For this review, take the finished solid that the model builds, in its own axes (mm). Face numbers are marked on the shaded views. A direction names the side the tool comes from. Round coordinates to 2 decimals unless told otherwise and drop trailing zeros. Write each loop counter-clockwise with the first axis right and the second up, starting at its lowest first coordinate (ties: lowest second). Pieces come first, ordered by that corner, then holes. Notation, with made-up numbers: M 33,-2.5 L 55,-2.5 A18 ccw 55,26.5 Z; hole C 64.25,-35.75 d5. An arc over 180 degrees is marked long. One line per question, with ' | ' between items.
```python
from build123d import *

# Parameters (mm, degrees)
EXTRUSION1_DEPTH = 28.5


with BuildPart() as part:
    # Esquisse1 → Révolution1 (revolve)
    with BuildSketch(Plane.XY):
        Polygon((-2.5, 19.6), (-2.5, 26), (-0.5, 26), (-0.5, 23.6), (2.5, 23.6), (2.5, 30), (20, 30), (20, 23.6), (23, 23.6), (23, 26), (25, 26), (25, 4), (10, 4), (10, 19.6), align=None)
    revolve(axis=Axis((10, 0, 0), (1, 0, 0)))

    # Esquisse2 → Extrusion1 (cut, through all)
    with BuildSketch(Plane(origin=(25, 0, 0), x_dir=(0, 0, -1), z_dir=(1, 0, 0))):
        with BuildLine():
            Line((17.944358445, 3), (-17.944358445, 3))
            ThreePointArc((-17.944358445, 3), (-19.127003214, 3.577312972), (-19.399306427, 4.864864865))
            ThreePointArc((-19.399306427, 4.864864865), (0, 20), (19.399306427, 4.864864865))
            ThreePointArc((19.399306427, 4.864864865), (19.127003214, 3.577312972), (17.944358445, 3))
        make_face()
    extrude(amount=-EXTRUSION1_DEPTH, mode=Mode.SUBTRACT)


solid = part.part
```
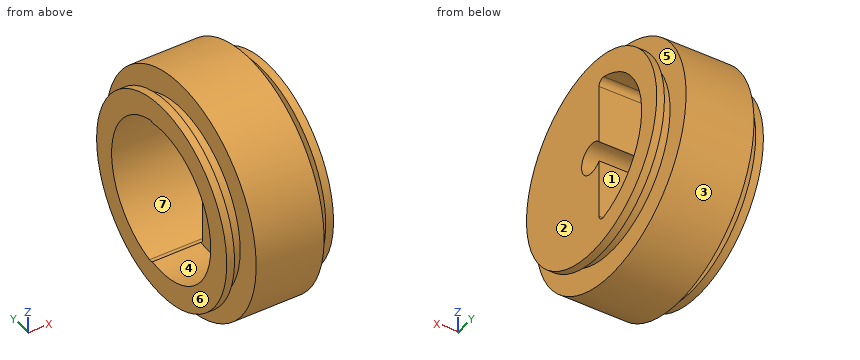
Item 1: Take a section at B-B (z = 0). Write out the cut boundary in (x, y), then the cut area to 3 significant figures.
Results:
outline: M -2.5,-26 L -0.5,-26 L -0.5,-23.6 L 2.5,-23.6 L 2.5,-30 L 20,-30 L 20,-23.6 L 23,-23.6 L 23,-26 L 25,-26 L 25,-4 L 10,-4 L 10,-19.6 L -2.5,-19.6 Z; M -2.5,20 L 25,20 L 25,26 L 23,26 L 23,23.6 L 20,23.6 L 20,30 L 2.5,30 L 2.5,23.6 L -0.5,23.6 L -0.5,26 L -2.5,26 Z | area: 686 mm2
Item 2: Take a section at D-D (z = -7). Write out the cut boundary in (x, y) (3 decimals), then the cut area to 3 significant figures.
Results:
outline: M -2.5,-25.04 L -0.5,-25.04 L -0.5,-22.538 L 2.5,-22.538 L 2.5,-29.172 L 20,-29.172 L 20,-22.538 L 23,-22.538 L 23,-25.04 L 25,-25.04 L 25,3 L 10,3 L 10,-18.307 L -2.5,-18.307 Z; M -2.5,18.735 L 25,18.735 L 25,25.04 L 23,25.04 L 23,22.538 L 20,22.538 L 20,29.172 L 2.5,29.172 L 2.5,22.538 L -0.5,22.538 L -0.5,25.04 L -2.5,25.04 Z | area: 793 mm2
Item 3: To check wall thickness, follow line 1 along X through (y, z) = (3, 25); line 2 along Z through (x, y) = (18.25, 0); line 3 along Z through (x, y) = (21.5, 0). State the ranges of each line that lie inside material, in increasing order. Write a range as from..to.
Results:
line 1: -2.5..-0.5, 2.5..20, 23..25 | line 2: -30..-4, 4..30 | line 3: -23.6..-4, 4..23.6
Item 4: Mouldability with a two-part tool opening along Z and no side actions: class the marked faces 1, 2, 3 and 4 as +Z half, -Z half, draft (parallel to the pull), parting line (faces both ways), or undercut.
Results:
face 1: undercut | face 2: draft | face 3: parting line | face 4: undercut
Item 5: Take a section at A-A (y = 0). Write out the cut boundary in (x, z).
Results:
outline: M -2.5,-26 L -0.5,-26 L -0.5,-23.6 L 2.5,-23.6 L 2.5,-30 L 20,-30 L 20,-23.6 L 23,-23.6 L 23,-26 L 25,-26 L 25,-4 L 10,-4 L 10,-19.6 L -2.5,-19.6 Z; M -2.5,19.6 L 10,19.6 L 10,4 L 25,4 L 25,26 L 23,26 L 23,23.6 L 20,23.6 L 20,30 L 2.5,30 L 2.5,23.6 L -0.5,23.6 L -0.5,26 L -2.5,26 Z
Item 6: Insertion check: pin 1 Ø4 at (x, z) = (8, -15.5) entering from -Y; pin 2 Ø4 at (x, y) = (3.5, 23.5) entering from +Z; pin 3 Ø1.5 at (x, z) = (2, 12) entering from +Y. Each pin has a flat end and moves straight along its axis. Give the tip position at first contact, or say it passes through.
Results:
pin 1: y = -26.79 | pin 2: z = 20.92 | pin 3: y = 27.73
Item 7: Take a section at C-C (x = 21). Write out the cut boundary in (y, z).
Results:
outline: C 0,0 d47.2; hole M 3,-17.94 A1.5 ccw 4.86,-19.4 A20 ccw 4.86,19.4 A1.5 ccw 3,17.94 L 3,2.65 A4 ccw long 3,-2.65 Z
Item 8: Machinability: for the marked faces 5, 6 and 7, which of the approach directions +Z, -Z, +X, -X, +Y, -Y give a long, thin tool a straight path to every point of the face, cutting with its end or side? Answer none if there is none.
Results:
face 5: none | face 6: +Z, -Z, -X, +Y, -Y | face 7: +X, -X
